Verification items for the finished model (mm, model axes). Face numbers are marked on the shaded views. A direction names the side the tool comes from. Coordinates: 2 decimals unless noted, no trailing zeros. Order: outer loops, then holes, each group sorted by start corner. A loop starts at its lowest first (then second) coordinate and runs counter-clockwise, first axis right, second up. Notation, with made-up numbers: (41, 37) - (59, 37) arc R7 ccw to (59, 49) - close; hole circle Ø9 at (-6.75, 26). An arc over 180 degrees is marked (long way). Answer as CSV lines item,"result". Start each with the question number.
1. Go/stop test with flat-tipped pins: pin 1 (3 mm diameter, centred on x = 133, z = -42, fed in from +Y); pin 2 (1.4 mm diameter, centred on y = 19.5, z = -71.5, fed in from +X) (3 decimals); pin 3 (3.5 mm diameter, centred on x = 117.475, z = -62.865, fed in from -Y); pin 4 (4.5 mm diameter, centred on x = 115.5, z = -44, fed in from +Y). Record where each tip stops, or that it passes through.
2. Section check A-A (z = -39.37). Record the cut outline in (x, y) (1 decimal), and give its area (3 significant figures).
3. Section check B-B (x = 61). Record the cut outline in (y, z).
4. Material ranges on L1, parallel to Z at x = 6, y = 26; L2, parallel to X at y = 6, z = -39.5 (3 decimals); L3, parallel to Z at x = 48, y = 34.5, recorded low to high. Write a range as [from, to].
5. Set-up check for the marked faces 4 and 5: record each of +Z, -Z, +X, -X, +Y, -Y from which the full face is reachable in a straight line by a thin tool's end or side.
6. Section check C-C (y = 24). Count the separate pieces of the cut face and the enclosed holes in it, and give its area (3 significant figures).
7. Mould release check, pull along Z, two halves, no side actions. Record for the marked faces 1, 2 and 3: pulls with the +Z half, pulls with the -Z half, needs draft (parallel to the pull), parting line crosses it, or undercut.
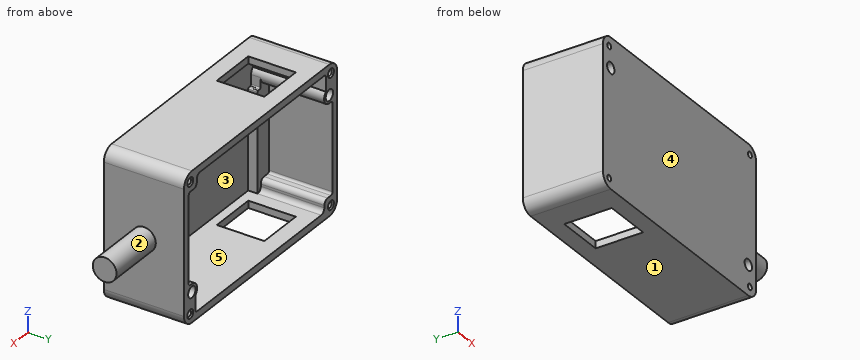
from build123d import *

# Parameters (mm, degrees)
BOSS_EXTRUDE1_DEPTH                               = 42.8625
CSK_FOR_0_FLAT_HEAD_MACHINE_SCREW_100_D           = 3.175
CSK_FOR_0_FLAT_HEAD_MACHINE_SCREW_100_CSINK_D     = 4.7625
CSK_FOR_0_FLAT_HEAD_MACHINE_SCREW_100_CSINK_ANGLE = 100
A_0_234_DIAMETER_HOLE1_D                          = 5.9436
A_0_234_DIAMETER_HOLE1_DEPTH                      = 42.8625
CUT_EXTRUDE1_DEPTH                                = 39.0525
BOSS_EXTRUDE2_DEPTH                               = 5.08
SKETCH12_W                                        = 25.4
SKETCH12_H                                        = 25.4
CUT_EXTRUDE2_DEPTH                                = 79.74
SKETCH13_R                                        = 6.35
BOSS_EXTRUDE3_DEPTH                               = 31.75


with BuildPart() as part:
    # Sketch1 → Boss-Extrude1 (new body)
    with BuildSketch(Plane(origin=(0, 0, 0), x_dir=(1, 0, 0), z_dir=(0, 1, 0))):
        with BuildLine():
            Line((6.35, 0), (117.475, 0))
            ThreePointArc((117.475, 0), (121.965128061, 1.859871939), (123.825, 6.35))
            Line((123.825, 6.35), (123.825, 72.39))
            ThreePointArc((123.825, 72.39), (121.965128061, 76.880128061), (117.475, 78.74))
            Line((117.475, 78.74), (6.35, 78.74))
            ThreePointArc((6.35, 78.74), (1.859871939, 76.880128061), (0, 72.39))
            Line((0, 72.39), (0, 6.35))
            ThreePointArc((0, 6.35), (1.859871939, 1.859871939), (6.35, 0))
        make_face()
    extrude(amount=BOSS_EXTRUDE1_DEPTH)

    # CSK for #0 Flat Head Machine Screw (100)1 (through all)
    with Locations(Plane(origin=(0, 42.8625, 0), x_dir=(1, 0, 0), z_dir=(0, 1, 0))):
        with Locations((5.08, 5.08), (5.08, 73.66), (118.745, 73.66), (118.745, 5.08)):
            CounterSinkHole(CSK_FOR_0_FLAT_HEAD_MACHINE_SCREW_100_D / 2, CSK_FOR_0_FLAT_HEAD_MACHINE_SCREW_100_CSINK_D / 2, counter_sink_angle=CSK_FOR_0_FLAT_HEAD_MACHINE_SCREW_100_CSINK_ANGLE)

    # A (0.234) Diameter Hole1
    with Locations(Plane(origin=(0, 42.8625, 0), x_dir=(1, 0, 0), z_dir=(0, 1, 0))):
        with Locations((6.35, 15.875), (117.475, 62.865)):
            Hole(A_0_234_DIAMETER_HOLE1_D / 2, depth=A_0_234_DIAMETER_HOLE1_DEPTH)

    # Sketch9 → Cut-Extrude1 (cut)
    with BuildSketch(Plane(origin=(0, 42.8625, 0), x_dir=(1, 0, 0), z_dir=(0, 1, 0))):
        with BuildLine():
            Line((5.08, 68.58), (7.880598047, 68.58))
            ThreePointArc((7.880598047, 68.58), (9.676649271, 69.323948776), (10.420598047, 71.12))
            Line((10.420598047, 71.12), (10.420598047, 72.39))
            ThreePointArc((10.420598047, 72.39), (11.164546822, 74.186051224), (12.960598047, 74.93))
            Line((12.960598047, 74.93), (61.9125, 74.93))
            Line((61.9125, 74.93), (113.404401953, 74.93))
            ThreePointArc((113.404401953, 74.93), (114.302427566, 74.558025612), (114.674401953, 73.66))
            Line((114.674401953, 73.66), (114.674401953, 66.05083079))
            ThreePointArc((114.674401953, 66.05083079), (113.505962063, 61.368468979), (117.475, 58.6232))
            Line((117.475, 58.6232), (118.745, 58.6232))
            ThreePointArc((118.745, 58.6232), (119.643025612, 58.251225612), (120.015, 57.3532))
            Line((120.015, 57.3532), (120.015, 11.43))
            ThreePointArc((120.015, 11.43), (119.643025612, 10.531974388), (118.745, 10.16))
            Line((118.745, 10.16), (115.944401953, 10.16))
            ThreePointArc((115.944401953, 10.16), (114.148350729, 9.416051224), (113.404401953, 7.62))
            Line((113.404401953, 7.62), (113.404401953, 6.35))
            ThreePointArc((113.404401953, 6.35), (112.660453178, 4.553948776), (110.864401953, 3.81))
            Line((110.864401953, 3.81), (61.9125, 3.81))
            Line((61.9125, 3.81), (10.420598047, 3.81))
            ThreePointArc((10.420598047, 3.81), (9.522572434, 4.181974388), (9.150598047, 5.08))
            Line((9.150598047, 5.08), (9.150598047, 12.68916921))
            ThreePointArc((9.150598047, 12.68916921), (10.319037937, 17.371531021), (6.35, 20.1168))
            Line((6.35, 20.1168), (5.08, 20.1168))
            ThreePointArc((5.08, 20.1168), (4.181974388, 20.488774388), (3.81, 21.3868))
            Line((3.81, 21.3868), (3.81, 67.31))
            ThreePointArc((3.81, 67.31), (4.181974388, 68.208025612), (5.08, 68.58))
        make_face()
    extrude(amount=-CUT_EXTRUDE1_DEPTH, mode=Mode.SUBTRACT)

    # Sketch11 → Boss-Extrude2 (add)
    with BuildSketch(Plane(origin=(0, 3.81, 0), x_dir=(1, 0, 0), z_dir=(0, 1, 0))):
        with BuildLine():
            Line((12.960598047, 74.93), (12.960598047, 22.225))
            ThreePointArc((12.960598047, 22.225), (12.774610853, 21.775987194), (12.325598047, 21.59))
            Line((12.325598047, 21.59), (11.2268, 21.59))
            ThreePointArc((11.2268, 21.59), (10.777787194, 21.404012806), (10.5918, 20.955))
            Line((10.5918, 20.955), (10.5918, 15.875))
            ThreePointArc((10.5918, 15.875), (9.349405544, 18.874405544), (6.35, 20.1168))
            Line((6.35, 20.1168), (5.08, 20.1168))
            ThreePointArc((5.08, 20.1168), (4.181974388, 20.488774388), (3.81, 21.3868))
            Line((3.81, 21.3868), (3.81, 67.31))
            ThreePointArc((3.81, 67.31), (4.181974388, 68.208025612), (5.08, 68.58))
            Line((5.08, 68.58), (7.880598047, 68.58))
            ThreePointArc((7.880598047, 68.58), (9.676649271, 69.323948776), (10.420598047, 71.12))
            Line((10.420598047, 71.12), (10.420598047, 72.39))
            ThreePointArc((10.420598047, 72.39), (11.164546822, 74.186051224), (12.960598047, 74.93))
        make_face()
        with BuildLine():
            Line((110.864401953, 3.81), (110.864401953, 56.515))
            ThreePointArc((110.864401953, 56.515), (111.050389147, 56.964012806), (111.499401953, 57.15))
            Line((111.499401953, 57.15), (112.5982, 57.15))
            ThreePointArc((112.5982, 57.15), (113.047212806, 57.335987194), (113.2332, 57.785))
            Line((113.2332, 57.785), (113.2332, 62.865))
            ThreePointArc((113.2332, 62.865), (114.475594456, 59.865594456), (117.475, 58.6232))
            Line((117.475, 58.6232), (118.745, 58.6232))
            ThreePointArc((118.745, 58.6232), (119.643025612, 58.251225612), (120.015, 57.3532))
            Line((120.015, 57.3532), (120.015, 11.43))
            ThreePointArc((120.015, 11.43), (119.643025612, 10.531974388), (118.745, 10.16))
            Line((118.745, 10.16), (115.944401953, 10.16))
            ThreePointArc((115.944401953, 10.16), (114.148350729, 9.416051224), (113.404401953, 7.62))
            Line((113.404401953, 7.62), (113.404401953, 6.35))
            ThreePointArc((113.404401953, 6.35), (112.660453178, 4.553948776), (110.864401953, 3.81))
        make_face()
    extrude(amount=BOSS_EXTRUDE2_DEPTH)

    # Sketch12 → Cut-Extrude2 (cut, through all)
    with BuildSketch(Plane(origin=(0, 0, -78.74), x_dir=(-1, 0, 0), z_dir=(0, 0, -1))):
        with Locations((-33.02, 21.43125)):
            Rectangle(SKETCH12_W, SKETCH12_H)
    extrude(amount=-CUT_EXTRUDE2_DEPTH, mode=Mode.SUBTRACT)

    # Sketch13 → Boss-Extrude3 (add)
    with BuildSketch(Plane(origin=(123.825, 0, 0), x_dir=(0, 0, -1), z_dir=(1, 0, 0))):
        with Locations((39.37, 21.43125)):
            Circle(SKETCH13_R)
    extrude(amount=BOSS_EXTRUDE3_DEPTH)


solid = part.part
Evaluation:
1,pin 1,"stops at y = 27.68"
1,pin 2,"stops at x = 123.825"
1,pin 3,"passes through"
1,pin 4,"stops at y = 8.89"
2,outline,"(0, 0) - (123.8, 0) - (123.8, 15.1) - (155.6, 15.1) - (155.6, 27.8) - (123.8, 27.8) - (123.8, 42.9) - (120, 42.9) - (120, 8.9) - (110.9, 8.9) - (110.9, 3.8) - (13, 3.8) - (13, 8.9) - (3.8, 8.9) - (3.8, 42.9) - (0, 42.9) - close"
2,area,"1,270 mm²"
3,outline,"(0, -78.74) - (42.86, -78.74) - (42.86, -74.93) - (3.81, -74.93) - (3.81, -3.81) - (42.86, -3.81) - (42.86, 0) - (0, 0) - close"
4,L1,"z = [-78.73, -74.95], [-72.37, -68.58], [-20.12, -18.83], [-12.92, -6.37], [-3.79, -0.01]"
4,L2,"x = [0, 12.961], [110.864, 123.825]"
4,L3,"z = [-78.74, -74.93], [-3.81, 0]"
5,face 4,"+Z, -Z, +X, -X, -Y"
5,face 5,"+Y"
6,separate pieces,"2"
6,enclosed holes,"6"
6,area,"1,810 mm²"
7,face 1,"pulls with the -Z half"
7,face 2,"parting line crosses it"
7,face 3,"undercut"
